Input: part model. Units: mm. Frame: model coordinates. Face numbers are marked on the shaded views. A direction names the side the tool comes from. Round coordinates to 2 decimals unless told otherwise and drop trailing zeros. Loops run counter-clockwise (first coordinate to the right, second up) from the corner with the lowest first, then second, coordinate; pieces in that order, holes last. Notation, with made-up numbers: M 86.25,9.25 L 141.25,9.25 A22 cw 141.25,44.25 Z; hole C 56,-22 d8. An arc over 180 degrees is marked long. Return JSON: item names as keys, results as strings. Group by question number.
1) Section C-C (x = 8.5). Output: boundary loops of the cut face in (y, z).
2) Mould query, pull axis X, two halves, no side actions, for the marked faces 1, 2 and 3. Classes: +X half, -X half, draft (parallel to the pull), parting line (faces both ways), or undercut.
3) Section A-A (z = -5). Output: boundary loops of the cut face in (x, y).
4) Section B-B (y = -20). Output: boundary loops of the cut face in (x, z), plus the area to 3 significant figures.
5) Section D-D (x = 28.5). Output: boundary loops of the cut face in (y, z).
6) Contact query for flat-ended pins moving along their axis: P1, Ø1, axis at x = 5, z = -21, coming from the -Y side; P2, Ø2, axis at x = -21.5, z = 1.5, coming from the +Y side; P3, Ø6, axis at x = -11.5, y = -38.5, coming from the +Z side. Output: stop coordinate, or through.
7) Material intervals for line 1 (X direction, y = -11, z = 0); line 2 (Z direction, x = 0, y = -21.5); line 3 (Y direction, x = 35.5, z = 12), sorted ascending. Write a range as from..to.
8) Access query for the marked faces 4, 5 and 6. Directions: +Z, -Z, +X, -X, +Y, -Y. A direction counts if a zero-diameter tool reaches every point of the face in a straight line with its end or side. Return the directions, or none.
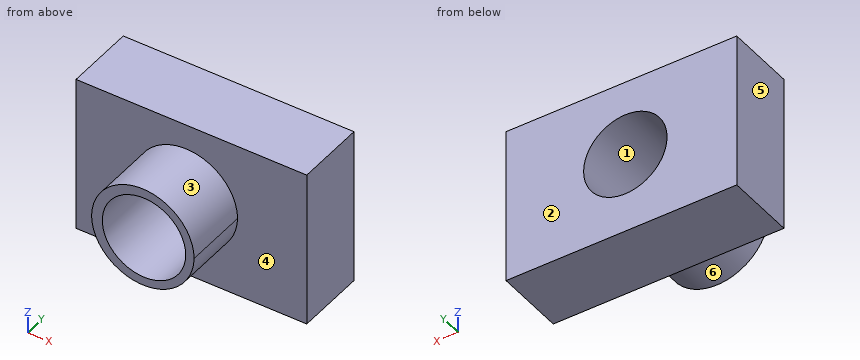
from build123d import *

# Parameters (mm, degrees)
F0_W     = 82.048778
F0_H     = 55.873601
F0_R     = 14.069549
F1_DEPTH = 25
F3_DEPTH = 48
F4_R     = 14.835097
F5_DEPTH = 49


with BuildPart() as f1:
    # F0 (on Front) → F1 (new body)
    with BuildSketch(Plane.XZ):
        with Locations((1.397414, -0.891356)):
            Rectangle(F0_W, F0_H)
        Circle(F0_R, mode=Mode.SUBTRACT)
    extrude(amount=F1_DEPTH)

    # F2 (on Front) → F3 (join)
    with BuildSketch(Plane.XZ):
        with BuildLine():
            ThreePointArc((-18.651316, 0), (-0.414473, -17.935191), (17.82237, 0))
            ThreePointArc((17.82237, 0), (-0.414473, 18.118096), (-18.651316, 0))
        make_face()
    extrude(amount=F3_DEPTH)

    # F4 (on Front) → F5 (cut)
    with BuildSketch(Plane.XZ):
        Circle(F4_R)
    extrude(amount=F5_DEPTH, mode=Mode.SUBTRACT)


solid = f1.part
Returned:
{
 "1": {"outline": "M -48,-15.61 L -25,-15.61 L -25,-28.83 L 0,-28.83 L 0,-12.16 L -48,-12.16 Z; M -48,12.16 L 0,12.16 L 0,27.05 L -25,27.05 L -25,15.79 L -48,15.79 Z"},
 "2": {"face 1": "undercut", "face 2": "draft", "face 3": "parting line"},
 "3": {"outline": "M -39.63,-25 L -17.87,-25 L -17.87,-48 L -13.97,-48 L -13.97,0 L -39.63,0 Z; M 13.97,-48 L 17.04,-48 L 17.04,-25 L 42.42,-25 L 42.42,0 L 13.97,0 Z"},
 "4": {"outline": "M -39.63,-28.83 L 42.42,-28.83 L 42.42,27.05 L -39.63,27.05 Z; hole C 0,0 d29.67", "area": "3,890 mm^2"},
 "5": {"outline": "M -25,-28.83 L 0,-28.83 L 0,27.05 L -25,27.05 Z"},
 "6": {"P1": "stops at y = -25", "P2": "stops at y = 0", "P3": "stops at z = 16.23"},
 "7": {"line 1": "x = -39.63..-14.84, 14.84..42.42", "line 2": "z = -28.83..-14.84, 14.84..27.05", "line 3": "y = -25..0"},
 "8": {"face 4": "-Y", "face 5": "+Z, -Z, -X, +Y, -Y", "face 6": "-Z, -Y"}
}
